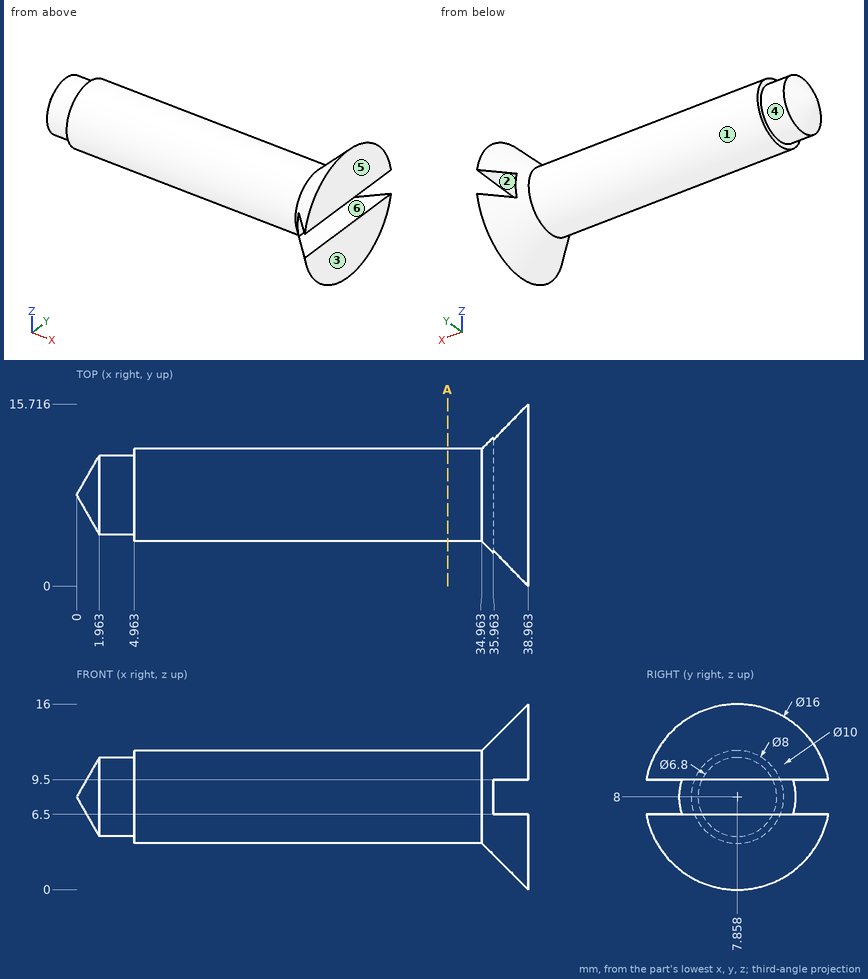
Job drawing, mm, ordinate dimensions from the low corner. One solid piece. A direction names the side the tool comes from. Round coordinates to 2 decimals unless told otherwise and drop trailing zeros. Loops run counter-clockwise (first coordinate to the right, second up) from the corner with the lowest first, then second, coordinate; pieces in that order, holes last. Notation, with made-up numbers: (55.5, 11) -> (87.5, 11) arc R21 ccw to (87.5, 43) -> close; hole circle Ø1 at (-16, 48.5). An arc over 180 degrees is marked (long way). Use a Markdown table: item, result.
1) Drop flat-ended pins along their axis: pin 1 Ø8 at (x, z) = (18.5, 4) entering from -Y; pin 2 Ø1.5 at (x, z) = (29, 14) entering from +Y; pin 3 Ø2.5 at (x, y) = (38, 6) entering from -Z; pin 4 Ø3 at (x, y) = (14.5, 11.5) entering from +Z. Give the stop position or say it passes through.
The answers:
| item | result |
|---|---|
| pin 1 | stops at y = 3.86 |
| pin 2 | passes through |
| pin 3 | stops at z = 0.07 |
| pin 4 | stops at z = 11.38 |
2) Pull direction Z, two halves, no side cores. Call the marked faces 1, 2 and 3: pulls with the +Z half, pulls with the -Z half, needs draft (parallel to the pull), parting line crosses it, or undercut.
The answers:
| item | result |
|---|---|
| face 1 | parting line crosses it |
| face 2 | undercut |
| face 3 | needs draft |
3) Probe line 1 (X direction, y = 8.5, z = 4.25); line 2 (Z direction, x = 21.5, y = 7.75); line 3 (Z direction, x = 16.5, y = 6.5). List the from-to ranges inside material, lowest first. Write a range as [from, to].
The answers:
| item | result |
|---|---|
| line 1 | x = [4.96, 38.96] |
| line 2 | z = [4, 12] |
| line 3 | z = [4.24, 11.76] |
4) Cut at A-A, the plane x = 32. List the corners of the cut face in (y, z), and give its area (3 significant figures).
The answers:
| item | result |
|---|---|
| outline | circle Ø8 at (7.86, 8) |
| area | 50.3 mm2 |
5) Tool access for the marked faces 4, 5 and 6: list every direction of +Z, -Z, +X, -X, +Y, -Y with a clear straight run to the whole face (end or side of a thin tool).
The answers:
| item | result |
|---|---|
| face 4 | -X |
| face 5 | +Z, -Z, +X, +Y, -Y |
| face 6 | +X, +Y, -Y |
